from build123d import *

# Parameters (mm, degrees)
EXTRUDE_1_DEPTH     = 15
EXTRUDE_START       = -5
SKETCH_2_R          = 15.1
EXTRUDE_2_DEPTH     = 5
CUT_EXTRUDE_START   = -15
SKETCH_4_W          = 4
SKETCH_4_H          = 29.19111141
CUT_EXTRUDE_1_DEPTH = 15
SKETCH_7_R          = 25
EXTRUDE_3_DEPTH     = 3
SKETCH_3_R          = 1.630422744
CUT_EXTRUDE_2_DEPTH = 9
SKETCH_8_R          = 1
CUT_EXTRUDE_3_DEPTH = 10


with BuildPart() as part:
    # 草图1 → 凸台-拉伸1 (new body)
    with BuildSketch(Plane.XY):
        with BuildLine():
            Line((13.379461873, 7), (20, 7))
            Line((20, 7), (22, 7))
            Line((22, 7), (22, 10))
            Line((22, 10), (11.314150432, 10))
            ThreePointArc((11.314150432, 10), (12.437589082, 8.562498341), (13.379461873, 7))
        make_face()
        with BuildLine():
            Line((6.812488532, 10), (11.314150432, 10))
            ThreePointArc((11.314150432, 10), (0, 15.1), (-11.314150432, 10))
            Line((-11.314150432, 10), (-6.812488532, 10))
            ThreePointArc((-6.812488532, 10), (0, 12.1), (6.812488532, 10))
        make_face()
        with BuildLine():
            Line((9.86965045, 7), (13.379461873, 7))
            ThreePointArc((13.379461873, 7), (12.437589082, 8.562498341), (11.314150432, 10))
            Line((11.314150432, 10), (6.812488532, 10))
            ThreePointArc((6.812488532, 10), (8.474871105, 8.636351067), (9.86965045, 7))
        make_face()
        with BuildLine():
            Line((-13.379461873, 7), (-9.86965045, 7))
            ThreePointArc((-9.86965045, 7), (-8.474871105, 8.636351067), (-6.812488532, 10))
            Line((-6.812488532, 10), (-11.314150432, 10))
            ThreePointArc((-11.314150432, 10), (-12.437589082, 8.562498341), (-13.379461873, 7))
        make_face()
        with BuildLine():
            ThreePointArc((-13.379461873, 7), (-12.437589082, 8.562498341), (-11.314150432, 10))
            Line((-11.314150432, 10), (-22, 10))
            Line((-22, 10), (-22, 7))
            Line((-22, 7), (-20, 7))
            Line((-20, 7), (-13.379461873, 7))
        make_face()
        with BuildLine():
            Line((-22, -10), (-11.314150432, -10))
            ThreePointArc((-11.314150432, -10), (-12.437589082, -8.562498341), (-13.379461873, -7))
            Line((-13.379461873, -7), (-20, -7))
            Line((-20, -7), (-22, -7))
            Line((-22, -7), (-22, -10))
        make_face()
        with BuildLine():
            ThreePointArc((11.314150432, -10), (12.437589082, -8.562498341), (13.379461873, -7))
            Line((13.379461873, -7), (9.86965045, -7))
            ThreePointArc((9.86965045, -7), (8.474871105, -8.636351067), (6.812488532, -10))
            Line((6.812488532, -10), (11.314150432, -10))
        make_face()
        with BuildLine():
            ThreePointArc((-6.812488532, -10), (-8.474871105, -8.636351067), (-9.86965045, -7))
            Line((-9.86965045, -7), (-13.379461873, -7))
            ThreePointArc((-13.379461873, -7), (-12.437589082, -8.562498341), (-11.314150432, -10))
            Line((-11.314150432, -10), (-6.812488532, -10))
        make_face()
        with BuildLine():
            ThreePointArc((-11.314150432, -10), (0, -15.1), (11.314150432, -10))
            Line((11.314150432, -10), (6.812488532, -10))
            ThreePointArc((6.812488532, -10), (0, -12.1), (-6.812488532, -10))
            Line((-6.812488532, -10), (-11.314150432, -10))
        make_face()
        with BuildLine():
            Line((22, -7), (20, -7))
            Line((20, -7), (13.379461873, -7))
            ThreePointArc((13.379461873, -7), (12.437589082, -8.562498341), (11.314150432, -10))
            Line((11.314150432, -10), (22, -10))
            Line((22, -10), (22, -7))
        make_face()
    extrude(amount=EXTRUDE_1_DEPTH)

    # 草图2 → 凸台-拉伸2 (add)
    with BuildSketch(Plane.XY.offset(EXTRUDE_START)):
        with Locations(Location((0, 0, 0), (0, 0, 152.381887639))):
            Circle(SKETCH_2_R)
    extrude(amount=EXTRUDE_2_DEPTH)

    # 草图4 → 切除-拉伸1 (cut)
    with BuildSketch(Plane.XY.offset(15).offset(CUT_EXTRUDE_START)):
        with Locations((0, 14.595555705)):
            Rectangle(SKETCH_4_W, SKETCH_4_H)
        with BuildLine():
            Line((-2, -14.96696362), (-2, -29.19111141))
            Line((-2, -29.19111141), (2, -29.19111141))
            Line((2, -29.19111141), (2, -14.96696362))
            ThreePointArc((2, -14.96696362), (0, -15.1), (-2, -14.96696362))
        make_face()
        with BuildLine():
            Line((-2, -11.933566106), (-2, -14.96696362))
            ThreePointArc((-2, -14.96696362), (0, -15.1), (2, -14.96696362))
            Line((2, -14.96696362), (2, -11.933566106))
            ThreePointArc((2, -11.933566106), (0, -12.1), (-2, -11.933566106))
        make_face()
    extrude(amount=CUT_EXTRUDE_1_DEPTH, mode=Mode.SUBTRACT)

    # 草图7 → 凸台-拉伸3 (add)
    with BuildSketch(Plane(origin=(0, 0, -5), x_dir=(-1, 0, 0), z_dir=(0, 0, -1))):
        Circle(SKETCH_7_R)
    extrude(amount=EXTRUDE_3_DEPTH)

    # 草图3 → 切除-拉伸2 (cut)
    with BuildSketch(Plane(origin=(0, 0, -5), x_dir=(-1, 0, 0), z_dir=(0, 0, -1))):
        with Locations((-12.914505057, 17.775291273)):
            Circle(SKETCH_3_R)
        with Locations((12.914505057, 17.775291273)):
            Circle(SKETCH_3_R)
        with Locations((20.89610813, -6.789557106)):
            Circle(SKETCH_3_R)
        with Locations((0, -21.971468333)):
            Circle(SKETCH_3_R)
        with Locations((-20.89610813, -6.789557106)):
            Circle(SKETCH_3_R)
    extrude(amount=CUT_EXTRUDE_2_DEPTH, mode=Mode.SUBTRACT)

    # 草图8 → 切除-拉伸3 (cut)
    with BuildSketch(Plane.XY):
        with Locations((-3, 7.95298686)):
            Circle(SKETCH_8_R)
        with Locations((0, 7.95298686)):
            Circle(SKETCH_8_R)
        with Locations((-1.5, 5.354910649)):
            Circle(SKETCH_8_R)
        with Locations((1.5, 5.354910649)):
            Circle(SKETCH_8_R)
        with Locations((3, 7.95298686)):
            Circle(SKETCH_8_R)
        with Locations((6.636688994, 5.310777645)):
            Circle(SKETCH_8_R)
        with Locations((7.563739977, 2.457608096)):
            Circle(SKETCH_8_R)
        with Locations((8.490790961, -0.395561453)):
            Circle(SKETCH_8_R)
        with Locations((5.556348158, 0.228173619)):
            Circle(SKETCH_8_R)
        with Locations((4.629297175, 3.081343168)):
            Circle(SKETCH_8_R)
        with Locations((7.101699371, -4.670745769)):
            Circle(SKETCH_8_R)
        with Locations((4.674648388, -6.434101526)):
            Circle(SKETCH_8_R)
        with Locations((2.247597405, -8.197457283)):
            Circle(SKETCH_8_R)
        with Locations((1.934012015, -5.213891597)):
            Circle(SKETCH_8_R)
        with Locations((4.361062998, -3.45053584)):
            Circle(SKETCH_8_R)
        with Locations((-2.247597405, -8.197457283)):
            Circle(SKETCH_8_R)
        with Locations((-4.674648388, -6.434101526)):
            Circle(SKETCH_8_R)
        with Locations((-7.101699371, -4.670745769)):
            Circle(SKETCH_8_R)
        with Locations((-4.361062998, -3.45053584)):
            Circle(SKETCH_8_R)
        with Locations((-1.934012015, -5.213891597)):
            Circle(SKETCH_8_R)
        with Locations((-8.490790961, -0.395561453)):
            Circle(SKETCH_8_R)
        with Locations((-7.563739977, 2.457608096)):
            Circle(SKETCH_8_R)
        with Locations((-6.636688994, 5.310777645)):
            Circle(SKETCH_8_R)
        with Locations((-4.629297175, 3.081343168)):
            Circle(SKETCH_8_R)
        with Locations((-5.556348158, 0.228173619)):
            Circle(SKETCH_8_R)
    extrude(amount=-CUT_EXTRUDE_3_DEPTH, mode=Mode.SUBTRACT)


solid = part.part
CAD build for the part. Positions are in the model's coordinates, mm. A direction names the side the tool comes from. Round coordinates to 2 decimals unless told otherwise and drop trailing zeros. Loops run counter-clockwise (first coordinate to the right, second up) from the corner with the lowest first, then second, coordinate; pieces in that order, holes last. Notation, with made-up numbers: M -35,-10 L -7,-10 A21 cw -7,6 Z; hole C 74.25,21.25 d5. An arc over 180 degrees is marked long. One line per question, with ' | ' between items. Start each with the question number.
Item 1: Wall check: line 1 (Y direction, x = 0, z = -5.5); line 2 (Y direction, x = -18.5, z = 5); line 3 (Y direction, x = 0, z = -2). Give the ranges that are in metal, low to high.
Item 2: Cut at A-A, the plane z = 7.75. Write the cut outline in (x, y), plus the area to 3 significant figures.
Item 3: Pin check, flat tips, straight feed: pin 1 Ø1.5 at (y, z) = (-14, 6.5) entering from -X; pin 2 Ø10 at (y, z) = (-20, -5) entering from +X; pin 3 Ø1.2 at (x, y) = (-4.67, -6.43) entering from +Z; pin 4 Ø1.5 at (y, z) = (-0.5, -3) entering from +X. Stop position of each tip, or through.
Item 4: Two-plate mould, pull along Y, no slides. Class faces 1 (the flat face through (0, 0, 0)), 2 (the cylindrical face through (-23.846, 7.509, -6.479)), 3 (the flat face through (12, -9, 15)): pulls with the +Y half, pulls with the -Y half, needs draft (parallel to the pull), parting line crosses it, or undercut.
Item 5: Which spindle directions (+Z, -Z, +X, -X, +Y, -Y) get a long thin tool onto all of the face, cutting with end or side? Do faces 4 (the flat face through (-17, -8, 0)), 5 (the cylindrical face through (22.525, -6.718, -6.479)), 6 (the cylindrical face through (-1.4, -4.37, -3.94)), 7 (the flat face through (2, -13, 7)), 8 (the flat face through (17, 9, 0)). Say none if no direction does.
Item 6: Cut at B-B, the plane y = 17. Write the cut outline in (x, z).
Item 7: Cut at D-D, the plane y = -11. Write the cut outline in (x, z).
Item 8: Cut at C-C, the plane x = 12. Write the cut outline in (y, z).
Responses:
1) line 1: y = -25 to -23.6, -20.34 to 6.95, 8.95 to 25 | line 2: y = -10 to -7, 7 to 10 | line 3: y = -15.1 to 6.95, 8.95 to 15.1
2) outline: M -22,-10 L -11.31,-10 A15.1 ccw -2,-14.97 L -2,-11.93 A12.1 cw -9.87,-7 L -22,-7 Z; M -22,7 L -9.87,7 A12.1 cw -2,11.93 L -2,14.97 A15.1 ccw -11.31,10 L -22,10 Z; M 2,-14.97 A15.1 ccw 11.31,-10 L 22,-10 L 22,-7 L 9.87,-7 A12.1 cw 2,-11.93 Z; M 2,11.93 A12.1 cw 9.87,7 L 22,7 L 22,10 L 11.31,10 A15.1 ccw 2,14.97 Z | area: 259 mm²
3) pin 1: stops at x = -7.24 | pin 2: stops at x = 20 | pin 3: passes through | pin 4: stops at x = 15.1
4) face 1: undercut | face 2: parting line crosses it | face 3: needs draft
5) face 4: -X, -Y | face 5: -Z | face 6: +Z, -Z | face 7: +Z, +Y, -Y | face 8: +X, +Y
6) outline: M -18.33,-8 L -14.35,-8 L -14.35,-5 L -18.33,-5 Z; M -11.48,-8 L 11.48,-8 L 11.48,-5 L -11.48,-5 Z; M 14.35,-8 L 18.33,-8 L 18.33,-5 L 14.35,-5 Z
7) outline: M -22.45,-8 L 22.45,-8 L 22.45,-5 L 10.34,-5 L 10.34,15 L 5.04,15 L 5.04,0 L -5.04,0 L -5.04,15 L -10.34,15 L -10.34,-5 L -22.45,-5 Z
8) outline: M -21.93,-8 L 16.43,-8 L 16.43,-5 L 9.17,-5 L 9.17,0 L 10,0 L 10,15 L 7,15 L 7,0 L -7,0 L -7,15 L -10,15 L -10,0 L -9.17,0 L -9.17,-5 L -21.93,-5 Z; M 19.13,-8 L 21.93,-8 L 21.93,-5 L 19.13,-5 Z
